from build123d import *

# Parameters (mm, degrees)
F1_DEPTH = 3
F2_DEPTH = 18


with BuildPart() as f1:
    # F0 (on Top) → F1 (new body)
    with BuildSketch(Plane.XY):
        with BuildLine():
            Line((8.2505, 5), (-8.2505, 5))
            Line((-8.2505, 5), (-8.2505, 3.75))
            ThreePointArc((-8.2505, 3.75), (-7.3666165235, 3.3838834765), (-7.0005, 2.5))
            ThreePointArc((-7.0005, 2.5), (-7.3666165235, 1.6161165235), (-8.2505, 1.25))
            Line((-8.2505, 1.25), (-8.2505, 0))
            Line((-8.2505, 0), (8.2505, 0))
            ThreePointArc((8.2505, 0), (5.7505, 2.5), (8.2505, 5))
        make_face()
        with BuildLine():
            ThreePointArc((10.7505, 2.5), (10.018266953, 4.267766953), (8.2505, 5))
            Line((8.2505, 5), (8.2505, 4))
            ThreePointArc((8.2505, 4), (9.3111601718, 3.5606601718), (9.7505, 2.5))
            ThreePointArc((9.7505, 2.5), (9.3111601718, 1.4393398282), (8.2505, 1))
            Line((8.2505, 1), (8.2505, 0))
            ThreePointArc((8.2505, 0), (10.018266953, 0.732233047), (10.7505, 2.5))
        make_face()
        with BuildLine():
            Line((8.2505, 4), (8.2505, 5))
            ThreePointArc((8.2505, 5), (5.7505, 2.5), (8.2505, 0))
            Line((8.2505, 0), (8.2505, 1))
            ThreePointArc((8.2505, 1), (6.7505, 2.5), (8.2505, 4))
        make_face()
        with BuildLine():
            ThreePointArc((-7.0005, 2.5), (-7.3666165235, 3.3838834765), (-8.2505, 3.75))
            Line((-8.2505, 3.75), (-8.2505, 1.25))
            ThreePointArc((-8.2505, 1.25), (-7.3666165235, 1.6161165235), (-7.0005, 2.5))
        make_face()
        with BuildLine():
            Line((-8.2505, 1.25), (-8.2505, 3.75))
            ThreePointArc((-8.2505, 3.75), (-9.5005, 2.5), (-8.2505, 1.25))
        make_face()
    extrude(amount=F1_DEPTH)

    # F0 (on Top) → F2 (join)
    with BuildSketch(Plane.XY):
        with BuildLine():
            ThreePointArc((-7.0005, 2.5), (-7.3666165235, 3.3838834765), (-8.2505, 3.75))
            Line((-8.2505, 3.75), (-8.2505, 1.25))
            ThreePointArc((-8.2505, 1.25), (-7.3666165235, 1.6161165235), (-7.0005, 2.5))
        make_face()
        with BuildLine():
            Line((-8.2505, 1.25), (-8.2505, 3.75))
            ThreePointArc((-8.2505, 3.75), (-9.5005, 2.5), (-8.2505, 1.25))
        make_face()
    extrude(amount=F2_DEPTH)


solid = f1.part
Design review of the part built by this model. Coordinates are the model's own, in mm. A direction names the side the tool comes from. Coordinates: 2 decimals unless noted, no trailing zeros. Order: outer loops, then holes, each group sorted by start corner. A loop starts at its lowest first (then second) coordinate and runs counter-clockwise, first axis right, second up.
Item 1: For line 1 (X direction, y = 2.55, z = 17); line 2 (Z direction, x = -2.25, y = 1.1); line 3 (X direction, y = 1.45, z = 16), list the stretches that pass through material, from the lowest coordinate up.
Item 2: For pin 1 Ø4 at (x, z) = (7.5, 4) entering from -Y; pin 2 Ø0.6 at (y, z) = (0.5, 1) entering from -X; pin 3 Ø2 at (x, y) = (-6, 2) entering from +Z, all flat-tipped, find the tip position at first contact; note any pin that passes through.
Item 3: For faces 1 (the flat face through (0, 3, 0)), 2 (the flat face through (-8.25, 1, 1)), 3 (the flat face through (-8.25, 4, 1)), 4 (the flat face through (0, 5, 1)), 5 (the cylindrical face through (-9.5, 2.55, 8.87)), list the 3-axis set-ups (+Z, -Z, +X, -X, +Y, -Y) from which the entire face can be reached by the end or side of a thin tool; tool diameter is ignored.
Item 4: Take a section at B-B, the plane x = 3.5. Write out the cut boundary in (y, z), then the cut area to 3 significant figures.
Item 5: Take a section at A-A, the plane z = 11.5. Write out the cut boundary in (x, y), then the cut area to 3 significant figures.
The answers:
1. line 1: x = -9.5 to -7
1. line 2: z = 0 to 3
1. line 3: x = -8.93 to -7.57
2. pin 1: stops at y = 0
2. pin 2: stops at x = -8.25
2. pin 3: stops at z = 3
3. face 1: -Z, +X, -X, +Y, -Y
3. face 2: +Z, -Z, -X, -Y
3. face 3: +Z, -Z, -X, +Y
3. face 4: +Z, -Z, +X, -X, +Y
3. face 5: +Z
4. outline: (0, 0) - (5, 0) - (5, 3) - (0, 3) - close
4. area: 15.0 mm2
5. outline: circle Ø2.5 at (-8.25, 2.5)
5. area: 4.91 mm2
